```python
from build123d import *

# Parameters (mm, degrees)
CROQUIS1_R              = 15
CROQUIS1_R_2            = 5
SALIENTE_EXTRUIR1_DEPTH = 9
CROQUIS2_R              = 13.5
CROQUIS2_R_2            = 13.2
CROQUIS2_R_3            = 6.8
CROQUIS2_R_4            = 6.5
CORTAR_EXTRUIR1_DEPTH   = 0.3


with BuildPart() as part:
    # Croquis1 → Saliente-Extruir1 (new body)
    with BuildSketch(Plane.XY):
        Circle(CROQUIS1_R)
        Circle(CROQUIS1_R_2, mode=Mode.SUBTRACT)
    extrude(amount=SALIENTE_EXTRUIR1_DEPTH)

    # Croquis2 → Cortar-Extruir1 (cut)
    with BuildSketch(Plane.XY.offset(9)):
        Circle(CROQUIS2_R)
        Circle(CROQUIS2_R_2, mode=Mode.SUBTRACT)
        Circle(CROQUIS2_R_3)
        Circle(CROQUIS2_R_4, mode=Mode.SUBTRACT)
    cortar_extruir1 = extrude(amount=-CORTAR_EXTRUIR1_DEPTH, mode=Mode.SUBTRACT)

    # Simetría1: Cortar-Extruir1 across plane
    add(cortar_extruir1.mirror(Plane.XY.offset(4.5)), mode=Mode.SUBTRACT)


solid = part.part
```
Could you check a few things on this model? Use its own coordinates, in mm. A direction names the side the tool comes from. Coordinates: 2 decimals unless noted, no trailing zeros. Loops run counter-clockwise (first coordinate to the right, second up) from the corner with the lowest first, then second, coordinate; pieces in that order, holes last.
1) Imagine slicing it at A-A (z = 3.25). List the corners of the cut face in (x, y) for me, and give its area (3 significant figures).
Reported:
outline: circle Ø30 at (0, 0); hole circle Ø10 at (0, 0)
area: 628 mm2
2) Thinking about a two-plate mould opening in X: for faces 4 (the face through (-11.18, 7.85, 9)), 5 (the face through (-2.93, -13.18, 8.85)), 6 (the face through (-14.985, 0.66, 4.437)), which applies, released by +X, released by -X, zero draft, split by the parting line, or undercut?
Reported:
face 4: zero draft
face 5: undercut
face 6: split by the parting line
3) Which directions (+Z, -Z, +X, -X, +Y, -Y) give clear straight access to the entire face, cutting with the end or side of a thin tool? Please do faces 1 (the face through (3.14, -6.03, 0.15)), 2 (the face through (-9.73, 8.92, 8.85)), 3 (the face through (2, -5, 0)).
Reported:
face 1: -Z
face 2: +Z
face 3: -Z, +X, -X, +Y, -Y
4) Imagine slicing it at C-C (x = 12). List the corners of the cut face in (y, z) for me, and give its area (3 significant figures).
Reported:
outline: (-9, 0) - (-6.18, 0) - (-6.18, 0.3) - (-5.5, 0.3) - (-5.5, 0) - (5.5, 0) - (5.5, 0.3) - (6.18, 0.3) - (6.18, 0) - (9, 0) - (9, 9) - (6.18, 9) - (6.18, 8.7) - (5.5, 8.7) - (5.5, 9) - (-5.5, 9) - (-5.5, 8.7) - (-6.18, 8.7) - (-6.18, 9) - (-9, 9) - close
area: 161 mm2
5) Will these pins go through, and if not, where does the flat tip stop? pin 1 Ø4 at (x, z) = (10.5, 3.5) entering from +Y; pin 2 Ø5 at (y, z) = (4, 1.5) entering from -X; pin 3 Ø2 at (x, z) = (-6.5, 4.5) entering from -Y.
Reported:
pin 1: stops at y = 12.36
pin 2: stops at x = -14.92
pin 3: stops at y = -13.96
6) Imagine slicing it at B-B (y = 11.5). List the corners of the cut face in (x, z) for me, and give its area (3 significant figures).
Reported:
outline: (-9.63, 0) - (-7.07, 0) - (-7.07, 0.3) - (-6.48, 0.3) - (-6.48, 0) - (6.48, 0) - (6.48, 0.3) - (7.07, 0.3) - (7.07, 0) - (9.63, 0) - (9.63, 9) - (7.07, 9) - (7.07, 8.7) - (6.48, 8.7) - (6.48, 9) - (-6.48, 9) - (-6.48, 8.7) - (-7.07, 8.7) - (-7.07, 9) - (-9.63, 9) - close
area: 173 mm2
7) Please list where these lines run through material, in increasing order: line 1 along Y through (x, z) = (0, 0.25); line 2 along Y through (x, z) = (0, 2.75); line 3 along Y through (x, z) = (1.5, 6.75).
Reported:
line 1: y = -15 to -13.5, -13.2 to -6.8, -6.5 to -5, 5 to 6.5, 6.8 to 13.2, 13.5 to 15
line 2: y = -15 to -5, 5 to 15
line 3: y = -14.92 to -4.77, 4.77 to 14.92
